Work out the finished part from the listing and answer in its coordinate system (mm). Face numbers are marked on the shaded views. Give positions to 0.01 mm unless a question says otherwise; leave off trailing zeros. Order: outer loops, then holes, each group sorted by start corner. A loop starts at its lowest first (then second) coordinate and runs counter-clockwise, first axis right, second up. Notation, with made-up numbers: (-35, -23.75) - (9, -23.75) arc R9 ccw to (9, -8.75) - close; hole circle Ø1 at (69, -0.5). An arc over 180 degrees is marked (long way). Put each result on its own line as item: value.
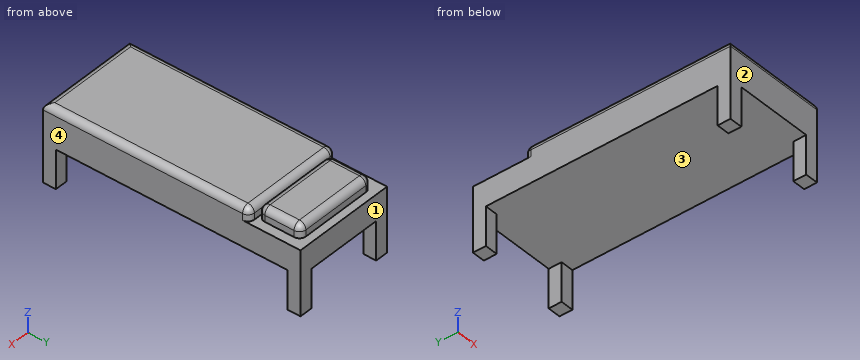
```python
from build123d import *

# Parameters (mm, degrees)
F0_W     = 800
F0_H     = 2000
F1_DEPTH = 200
F2_W     = 100
F2_H     = 100
F3_DEPTH = 300
F4_W     = 800
F4_H     = 1600
F5_DEPTH = 100
F6_R     = 50
F7_W     = 653.6028981209
F7_H     = 327.4476051331
F8_DEPTH = 100
F9_R     = 50


with BuildPart() as f1:
    # F0 (on Top) → F1 (new body)
    with BuildSketch(Plane.XY):
        Rectangle(F0_W, F0_H)
    extrude(amount=F1_DEPTH)

    # F2 (on face) → F3 (join)
    with BuildSketch(Plane(origin=(0, 0, 0), x_dir=(1, 0, 0), z_dir=(0, 0, -1))):
        with Locations((350, 950)):
            Rectangle(F2_W, F2_H)
        with Locations((-350, 950)):
            Rectangle(F2_W, F2_H)
        with Locations((-350, -950)):
            Rectangle(F2_W, F2_H)
        with Locations((350, -950)):
            Rectangle(F2_W, F2_H)
    extrude(amount=F3_DEPTH)

    # F4 (on face) → F5 (join)
    with BuildSketch(Plane.XY.offset(200)):
        with Locations((0, -200)):
            Rectangle(F4_W, F4_H)
    extrude(amount=F5_DEPTH)

    # F6
    f6_edges = [f1.edges().sort_by_distance(p)[0] for p in [
        (400, -200, 300),
        (0, -1000, 300),
        (-400, -200, 300),
        (0, 600, 300),
        (400, 600, 250),
        (-400, 600, 250),
    ]]
    fillet(f6_edges, radius=F6_R)

    # F7 (on face) → F8 (join)
    with BuildSketch(Plane.XY.offset(200)):
        with Locations((0, 775)):
            Rectangle(F7_W, F7_H)
    extrude(amount=F8_DEPTH)

    # F9
    f9_edges = [f1.edges().sort_by_distance(p)[0] for p in [
        (326.801449, 775, 300),
        (326.801449, 938.723803, 250),
        (0, 938.723803, 300),
        (-326.801449, 938.723803, 250),
        (-326.801449, 775, 300),
        (-326.801449, 611.276197, 250),
        (0, 611.276197, 300),
        (326.801449, 611.276197, 250),
    ]]
    fillet(f9_edges, radius=F9_R)


solid = f1.part
```
(1) Section A-A, the plane z = -49.5 is taken. Write down the section's boundary in (x, y).
Geometry check:
outline: (-400, -1000) - (-300, -1000) - (-300, -900) - (-400, -900) - close; (-400, 900) - (-300, 900) - (-300, 1000) - (-400, 1000) - close; (300, -1000) - (400, -1000) - (400, -900) - (300, -900) - close; (300, 900) - (400, 900) - (400, 1000) - (300, 1000) - close
(2) Section C-C, the plane y = 807.5 is taken. Write down the section's boundary in (x, z), then the cut area to 3 significant figures.
Geometry check:
outline: (-400, 0) - (400, 0) - (400, 200) - (326.8, 200) - (326.8, 250) arc R50 ccw to (276.8, 300) - (-276.8, 300) arc R50 ccw to (-326.8, 250) - (-326.8, 200) - (-400, 200) - close
area: 224,000 mm²
(3) Section B-B, the plane z = 218.5 is taken. Write down the section's boundary in (x, y).
Geometry check:
outline: (-400, -1000) - (400, -1000) - (400, 550) arc R50 ccw to (350, 600) - (-350, 600) arc R50 ccw to (-400, 550) - close; (-326.8, 661.28) arc R50 ccw to (-276.8, 611.28) - (276.8, 611.28) arc R50 ccw to (326.8, 661.28) - (326.8, 888.72) arc R50 ccw to (276.8, 938.72) - (-276.8, 938.72) arc R50 ccw to (-326.8, 888.72) - close
(4) Given pin 1 (25 mm diameter, centred on x = -126, z = 229, fed in from +Y); pin 2 (25 mm diameter, centred on y = 726, z = 216.5, fed in from -X); pin 3 (15 mm diameter, centred on y = 749.5, z = 232, fed in from +X), each flat-ended and moving along its own axis, determine where each tip first touches the part or whether it passes through.
Geometry check:
pin 1: stops at y = 938.72
pin 2: stops at x = -326.8
pin 3: stops at x = 326.8
(5) Straight lines are drawn through the part: line 1 (Y direction, x = 271, z = 233); line 2 (Z direction, x = -205.5, y = -771); line 3 (X direction, y = 673.5, z = 235.5). For each, find the intervals that lie inside material, in ascending order.
Geometry check:
line 1: y = -1000 to 600, 611.28 to 938.72
line 2: z = 0 to 300
line 3: x = -326.8 to 326.8
(6) Section D-D, the plane x = -113 is taken. Write down the section's boundary in (y, z), then the cut area to 3 significant figures.
Geometry check:
outline: (-1000, 0) - (1000, 0) - (1000, 200) - (938.72, 200) - (938.72, 250) arc R50 ccw to (888.72, 300) - (661.28, 300) arc R50 ccw to (611.28, 250) - (611.28, 200) - (600, 200) - (600, 250) arc R50 ccw to (550, 300) - (-950, 300) arc R50 ccw to (-1000, 250) - close
area: 591,000 mm²
(7) Determine the mould class of the marked faces 1, 2, 3 and 4 for opening direction Y: pulls with the +Y half, pulls with the -Y half, needs draft (parallel to the pull), parting line crosses it, or undercut.
Geometry check:
face 1: pulls with the +Y half
face 2: pulls with the -Y half
face 3: undercut
face 4: needs draft
